Can you work these out from the model? Positions are in its coordinate system, mm. A direction names the side the tool comes from. Round coordinates to 2 decimals unless told otherwise and drop trailing zeros. Loops run counter-clockwise (first coordinate to the right, second up) from the corner with the lowest first, then second, coordinate; pieces in that order, holes last.
from build123d import *

# Parameters (mm, degrees)
SKETCH1_R               = 5.325
BOSS_EXTRUDE1_DEPTH     = 14.4
SKETCH2_R               = 5.575
BOSS_EXTRUDE2_DEPTH     = 6.8
SKETCH3_R               = 6.225
BOSS_EXTRUDE3_DEPTH     = 24
FILLET1_R               = 5.325
CUT_EXTRUDE1_DEPTH      = 48
CUT_EXTRUDE1_DEPTH_BACK = 48
SKETCH5_R               = 3
CUT_EXTRUDE2_DEPTH      = 48
CHAMFER1_SIZE           = 0.5
SKETCH6_R               = 5
CUT_EXTRUDE3_DEPTH      = 32.5
CHAMFER2_SIZE           = 0.25


with BuildPart() as part:
    # Sketch1 → Boss-Extrude1 (new body)
    with BuildSketch(Plane.XY):
        Circle(SKETCH1_R)
    extrude(amount=BOSS_EXTRUDE1_DEPTH)

    # Sketch2 → Boss-Extrude2 (add)
    with BuildSketch(Plane.XY.offset(14.4)):
        Circle(SKETCH2_R)
    extrude(amount=BOSS_EXTRUDE2_DEPTH)

    # Sketch3 → Boss-Extrude3 (add)
    with BuildSketch(Plane.XY.offset(21.2)):
        Circle(SKETCH3_R)
    extrude(amount=BOSS_EXTRUDE3_DEPTH)

    # Fillet1
    fillet1_edges = [part.edges().sort_by_distance(p)[0] for p in [
        (-5.325, 0, 0),
    ]]
    fillet(fillet1_edges, radius=FILLET1_R)

    # Sketch4 → Cut-Extrude1 (cut, two sides)
    with BuildSketch(Plane(origin=(0, 0, 0), x_dir=(0, 0, -1), z_dir=(1, 0, 0))) as cut_extrude1_sk:
        Polygon((2.225204424, 1.725), (-11.35, 1.725), (-11.35, 16.315544117), (23.658725474, 16.315544117), (23.658725474, -14.317722388), (-11.35, -14.317722388), (-11.35, -1.725), (2.225204424, -1.725), align=None)
    extrude(amount=CUT_EXTRUDE1_DEPTH, mode=Mode.SUBTRACT)
    extrude(cut_extrude1_sk.sketch, amount=-CUT_EXTRUDE1_DEPTH_BACK, mode=Mode.SUBTRACT)

    # Sketch5 → Cut-Extrude2 (cut)
    with BuildSketch(Plane(origin=(0, 1.725, 0), x_dir=(1, 0, 0), z_dir=(0, 1, 0))):
        with Locations((0, -5.325)):
            Circle(SKETCH5_R)
    extrude(amount=-CUT_EXTRUDE2_DEPTH, mode=Mode.SUBTRACT)

    # Chamfer1
    chamfer1_edges = [part.edges().sort_by_distance(p)[0] for p in [
        (-6.225, 0, 21.2),
    ]]
    chamfer(chamfer1_edges, length=CHAMFER1_SIZE)

    # Sketch6 → Cut-Extrude3 (cut)
    with BuildSketch(Plane.XY.offset(45.2)):
        Circle(SKETCH6_R)
    extrude(amount=-CUT_EXTRUDE3_DEPTH, mode=Mode.SUBTRACT)

    # Chamfer2
    chamfer2_edges = [part.edges().sort_by_distance(p)[0] for p in [
        (-6.225, 0, 45.2),
    ]]
    chamfer(chamfer2_edges, length=CHAMFER2_SIZE)


solid = part.part
(1) Will these pins go through, and if not, where does the flat tip stop? P1, Ø1, axis at y = 1.5, z = 33, coming from the +X side; P2, Ø4, axis at x = -3.5, y = 0, coming from the -Z side; P3, Ø5, axis at x = 0.5, z = 7.5, coming from the +Y side (3 decimals).
Worked answers:
P1: stops at x = 6.14
P2: stops at z = 0.22
P3: stops at y = 1.725
(2) If we section it at A-A, the plane x = 0: List the corners of the cut face in (y, z) for me (3 decimals), then the cut area to 3 significant figures.
Worked answers:
outline: (-6.225, 21.7) - (-5.725, 21.2) - (-5.575, 21.2) - (-5.575, 14.4) - (-5.325, 14.4) - (-5.325, 11.35) - (-1.725, 11.35) - (-1.725, 8.325) - (1.725, 8.325) - (1.725, 11.35) - (5.325, 11.35) - (5.325, 14.4) - (5.575, 14.4) - (5.575, 21.2) - (5.725, 21.2) - (6.225, 21.7) - (6.225, 44.95) - (5.975, 45.2) - (5, 45.2) - (5, 12.7) - (-5, 12.7) - (-5, 45.2) - (-5.975, 45.2) - (-6.225, 44.95) - close; (-1.725, 0.287) arc R5.325 ccw to (1.725, 0.287) - (1.725, 2.325) - (-1.725, 2.325) - close
area: 99.9 mm2
(3) If we section it at C-C, the plane y = 0: List the corners of the cut face in (x, z) for me (3 decimals), then the cut area to 3 significant figures.
Worked answers:
outline: (-6.225, 21.7) - (-5.725, 21.2) - (-5.575, 21.2) - (-5.575, 14.4) - (-5.325, 14.4) - (-5.325, 5.325) arc R5.325 ccw to (5.325, 5.325) - (5.325, 14.4) - (5.575, 14.4) - (5.575, 21.2) - (5.725, 21.2) - (6.225, 21.7) - (6.225, 44.95) - (5.975, 45.2) - (5, 45.2) - (5, 12.7) - (-5, 12.7) - (-5, 45.2) - (-5.975, 45.2) - (-6.225, 44.95) - close; hole circle Ø6 at (0, 5.325)
area: 162 mm2
(4) If we mould it in two halves opening along X, with no side actions, what happens to faces 5 (the flat face through (0, 0, 12.7)), 6 (the flat face through (-4, -4, 45.2)), 7 (the cylindrical face through (-0.65, 0.024, 8.254)), 8 (the cylindrical face through (-4.588, 4.207, 33.162))? For each: released by +X, released by -X, zero draft, split by the parting line, or undercut.
Worked answers:
face 5: undercut
face 6: zero draft
face 7: undercut
face 8: split by the parting line
(5) If I drill on line 1 (Y direction, x = -0.25, z = 41.5); line 2 (Z direction, x = -1, y = -3.75); line 3 (Z direction, x = -4.25, y = 3.25), over which ranges is the centre line in solid material (lowest first)?
Worked answers:
line 1: y = -6.22 to -4.99, 4.99 to 6.22
line 2: z = 11.35 to 12.7
line 3: z = 14.4 to 45.2
(6) If we section it at D-D, the plane z = 32: List the corners of the cut face in (x, y) for me (3 decimals).
Worked answers:
outline: circle Ø12.45 at (0, 0); hole circle Ø10 at (0, 0)
(7) For faces 1 (the cylindrical face through (-1.08, -4.88, 29.18)), 2 (the flat face through (-2, 1.725, 8)), 3 (the flat face through (-1, -1.725, 8.4)), 4 (the cylindrical face through (5.32, 1.67, 17.75)), which set-ups out of +Z, -Z, +X, -X, +Y, -Y let a thin tool reach every point of the face, with its end or its side?
Worked answers:
face 1: +Z
face 2: -Z, +X, -X, +Y
face 3: -Z, +X, -X, -Y
face 4: -Z
(8) If we section it at B-B, the plane z = 6: List the corners of the cut face in (x, y) for me (3 decimals), then the cut area to 3 significant figures.
Worked answers:
outline: (-5.038, -1.725) - (-2.923, -1.725) - (-2.923, 1.725) - (-5.038, 1.725) arc R5.325 ccw to start; (2.923, -1.725) - (5.038, -1.725) arc R5.325 ccw to (5.038, 1.725) - (2.923, 1.725) - close
area: 15.9 mm2
